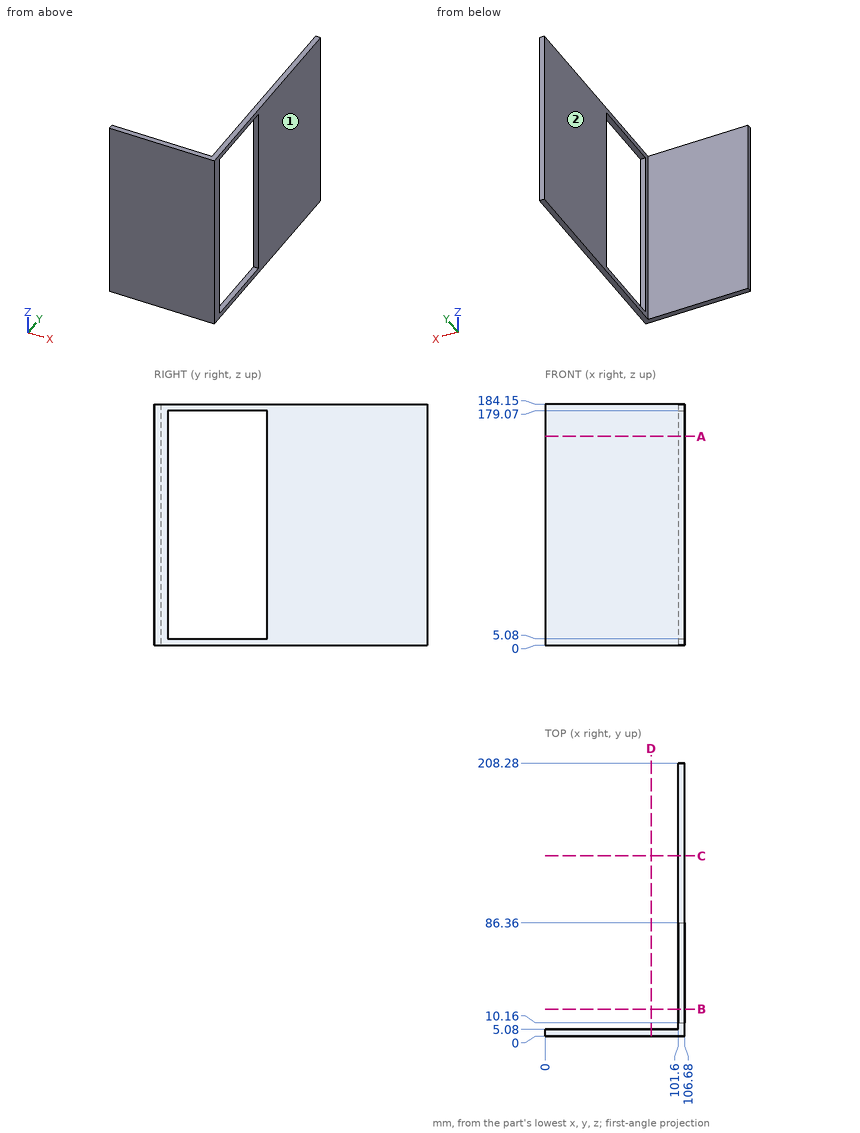
Input: dimensioned drawing with shaded views. Units: mm. Origin: part minimum x, y, z. A direction names the side the tool comes from. Round coordinates to 2 decimals unless told otherwise and drop trailing zeros. Order: outer loops, then holes, each group sorted by start corner. A loop starts at its lowest first (then second) coordinate and runs counter-clockwise, first axis right, second up.
Q1. Access query for the marked faces 1 and 2. Directions: +Z, -Z, +X, -X, +Y, -Y. A direction counts if a zero-diameter tool reaches every point of the face in a straight line with its end or side. Return the directions, or none.
Result sheet:
face 1: +Z, -Z, +X, +Y, -Y
face 2: +Z, -Z, -X, +Y
Q2. Material intervals for probe 1 along Y at (x, z) = (60, 138.5); probe 2 along X at (y, z) = (104, 12), sorted ascending.
Result sheet:
probe 1: y = 0 to 5.08
probe 2: x = 101.6 to 106.68
Q3. Section A-A, the plane z = 159.5. Output: boundary loops of the cut face in (x, y), and give its area (3 significant figures).
Result sheet:
outline: (0, 0) - (106.68, 0) - (106.68, 10.16) - (101.6, 10.16) - (101.6, 5.08) - (0, 5.08) - close; (101.6, 86.36) - (106.68, 86.36) - (106.68, 208.28) - (101.6, 208.28) - close
area: 1,190 mm2
Q4. Section C-C, the plane y = 137.5. Output: boundary loops of the cut face in (x, z), and give its area (3 significant figures).
Result sheet:
outline: (101.6, 0) - (106.68, 0) - (106.68, 184.15) - (101.6, 184.15) - close
area: 935 mm2
Q5. Pin query (flat end, axial travel): pin 1 (2.5 mm diameter, centred on x = 104, z = 50.5, fed in from -Y). Return the tip coordinate at first contact, or that it passes through.
Result sheet:
pin 1: stops at y = 0
Q6. Section D-D, the plane x = 81. Output: boundary loops of the cut face in (y, z).
Result sheet:
outline: (0, 0) - (5.08, 0) - (5.08, 184.15) - (0, 184.15) - close
Q7. Section B-B, the plane y = 20.5. Output: boundary loops of the cut face in (x, z).
Result sheet:
outline: (101.6, 0) - (106.68, 0) - (106.68, 5.08) - (101.6, 5.08) - close; (101.6, 179.07) - (106.68, 179.07) - (106.68, 184.15) - (101.6, 184.15) - close
